```python
from build123d import *

# Parameters (mm, degrees)
SKETCH1_W                       = 152.4
SKETCH1_H                       = 101.6
BOSS_EXTRUDE1_DEPTH             = 46.99
SKETCH2_R                       = 17.145
CUT_EXTRUDE1_DEPTH              = 190.093574983
SKETCH2_2_R                     = 25.4
SKETCH2_2_R_2                   = 17.145
CUT_EXTRUDE3_DEPTH              = 12.446
TAP_DRILL_FOR_1_2_13_TAP1_D     = 10.71626
TAP_DRILL_FOR_1_2_13_TAP1_DEPTH = 17.78
TAP_DRILL_FOR_1_2_13_TAP1_TIP   = 3.219489309


with BuildPart() as part:
    # Sketch1 → Boss-Extrude1 (new body)
    with BuildSketch(Plane.XY):
        with Locations((76.2, 50.8)):
            Rectangle(SKETCH1_W, SKETCH1_H)
    extrude(amount=BOSS_EXTRUDE1_DEPTH)

    # Sketch2 → Cut-Extrude1 (cut, through all)
    with BuildSketch(Plane(origin=(0, 0, 0), x_dir=(-1, 0, 0), z_dir=(0, 0, -1))):
        with Locations((-76.2, 50.8)):
            Circle(SKETCH2_R)
    extrude(amount=-CUT_EXTRUDE1_DEPTH, mode=Mode.SUBTRACT)

    # Sketch2<2> → Cut-Extrude3 (cut)
    with BuildSketch(Plane(origin=(0, 0, 0), x_dir=(-1, 0, 0), z_dir=(0, 0, -1))):
        with Locations((-76.2, 50.8)):
            Circle(SKETCH2_2_R)
        with Locations((-76.2, 50.8)):
            Circle(SKETCH2_2_R_2, mode=Mode.SUBTRACT)
    cut_extrude3 = extrude(amount=-CUT_EXTRUDE3_DEPTH, mode=Mode.SUBTRACT)

    # Mirror2: Cut-Extrude3 across plane
    add(cut_extrude3.mirror(Plane(origin=(0, 0, 23.495), x_dir=(1, 0, 0), z_dir=(0, 0, -1))), mode=Mode.SUBTRACT)

    # Tap Drill for 1/2-13 Tap1
    with Locations(Plane(origin=(0, 0, 0), x_dir=(-1, 0, 0), z_dir=(0, -1, 0))):
        with Locations((-66.653283, -23.495), (-28.553283, -23.495)):
            Hole(TAP_DRILL_FOR_1_2_13_TAP1_D / 2, depth=TAP_DRILL_FOR_1_2_13_TAP1_DEPTH)
            with Locations((0, 0, -(TAP_DRILL_FOR_1_2_13_TAP1_DEPTH + TAP_DRILL_FOR_1_2_13_TAP1_TIP / 2))):  # 118° drill point
                Cone(0, TAP_DRILL_FOR_1_2_13_TAP1_D / 2, TAP_DRILL_FOR_1_2_13_TAP1_TIP, mode=Mode.SUBTRACT)


solid = part.part
```
CAD build for the part. Positions are in the model's coordinates, mm. A direction names the side the tool comes from. Coordinates: 2 decimals unless noted, no trailing zeros. Order: outer loops, then holes, each group sorted by start corner. A loop starts at its lowest first (then second) coordinate and runs counter-clockwise, first axis right, second up. Notation, with made-up numbers: (10.5, 21) - (36.5, 21) arc R12 ccw to (36.5, 42) - close; hole circle Ø5 at (73.25, 73.25). An arc over 180 degrees is marked (long way). Use a Markdown table: item, result. Add a question column.
(1) Saw through at B-B (y = 50.8). Give the cut face in (x, z) (3 decimals), then the cut area to 3 significant figures.
(2) Pull direction Z, two halves, no side cores. Call faces 4 (the face through (75, 101.6, 23)), 5 (the face through (92, 29, 0)), 6 (the face through (24.604, 9.014, 19.874)): +Z half, -Z half, draft (parallel to the pull), parting line (faces both ways), or undercut.
(3) Saw through at C-C (z = 3.5). Give the cut face in (x, y).
(4) Flat gauge pin, fed straight in: pin 1 (1.5 mm diameter, centred on x = 52.5, y = 53.5, fed in from -Z). Where does the tip first touch, or does it go through?
(5) Drill centre lines: line 1 along Y through (x, z) = (77, 18.5); line 2 along X through (y, z) = (50, 37); line 3 along Y through (x, z) = (76.2, 38). Where is each one in solid material? Low to high. Write a range as [from, to].
(6) Saw through at D-D (y = 12). Give the cut face in (x, z) (3 decimals).
(7) Which spindle directions (+Z, -Z, +X, -X, +Y, -Y) get a long thin tool onto all of the face, cutting with end or side? Do faces 1 (the face through (79.507, 75.984, 40.854)), 2 (the face through (62.704, 9.014, 19.874)), 3 (the face through (59.6, 45.5, 12.446)). Say none if no direction does.
(8) Saw through at A-A (x = 76.2). Give the cut face in (y, z) (3 decimals).
Solved:
| question | item | result |
|---|---|---|
| 1 | outline | (0, 0) - (50.8, 0) - (50.8, 12.446) - (59.055, 12.446) - (59.055, 34.544) - (50.8, 34.544) - (50.8, 46.99) - (0, 46.99) - close; (93.345, 12.446) - (101.6, 12.446) - (101.6, 0) - (152.4, 0) - (152.4, 46.99) - (101.6, 46.99) - (101.6, 34.544) - (93.345, 34.544) - close |
| 1 | area | 5,140 mm² |
| 2 | face 4 | draft |
| 2 | face 5 | -Z half |
| 2 | face 6 | undercut |
| 3 | outline | (0, 0) - (152.4, 0) - (152.4, 101.6) - (0, 101.6) - close; hole circle Ø50.8 at (76.2, 50.8) |
| 4 | pin 1 | stops at z = 12.45 |
| 5 | line 1 | y = [0, 33.67], [67.93, 101.6] |
| 5 | line 2 | x = [0, 50.81], [101.59, 152.4] |
| 5 | line 3 | y = [0, 25.4], [76.2, 101.6] |
| 6 | outline | (0, 0) - (152.4, 0) - (152.4, 46.99) - (0, 46.99) - close; hole circle Ø10.716 at (28.553, 23.495); hole circle Ø10.716 at (66.653, 23.495) |
| 7 | face 1 | +Z |
| 7 | face 2 | -Y |
| 7 | face 3 | -Z |
| 8 | outline | (0, 0) - (25.4, 0) - (25.4, 12.446) - (33.655, 12.446) - (33.655, 34.544) - (25.4, 34.544) - (25.4, 46.99) - (0, 46.99) - close; (67.945, 12.446) - (76.2, 12.446) - (76.2, 0) - (101.6, 0) - (101.6, 46.99) - (76.2, 46.99) - (76.2, 34.544) - (67.945, 34.544) - close |
